```python
from build123d import *

# Parameters (mm, degrees)
SKETCH_1_R           = 1.6
EXTRUDE_1_DEPTH      = 6
SKETCH_2_R           = 30
CUT_EXTRUDE_1_DEPTH  = 13
SKETCH_3_R           = 3.5
CUT_EXTRUDE_2_DEPTH  = 3
SKETCH_5_R           = 2
CUT_EXTRUDE_3_DEPTH  = 23.5
SKETCH_6_R           = 4
CUT_EXTRUDE_4_DEPTH  = 2
CUT_EXTRUDE_6_REACH  = 134
SKETCH_8_W           = 137
SKETCH_8_H           = 2
CUT_EXTRUDE_7_REACH  = 139
SKETCH_9_W           = 1
SKETCH_9_H           = 132
SKETCH_10_W          = 29.336996967
SKETCH_10_H          = 52.898776648
CUT_EXTRUDE_11_DEPTH = 10
SKETCH_11_W          = 8.60940703
SKETCH_11_H          = 108.550160487
CUT_EXTRUDE_12_DEPTH = 10


with BuildPart() as part:
    # 草图1 → 凸台-拉伸1 (new body)
    with BuildSketch(Plane.XY):
        with BuildLine():
            Line((68.5, 66), (20, 66))
            ThreePointArc((20, 66), (0, 46), (-20, 66))
            Line((-20, 66), (-68.5, 66))
            Line((-68.5, 66), (-68.5, 17.384653731))
            ThreePointArc((-68.5, 17.384653731), (-52.74289675, 12.562504398), (-45.954411074, -2.452684221))
            ThreePointArc((-45.954411074, -2.452684221), (-52.74289675, -17.46787284), (-68.5, -22.290022173))
            Line((-68.5, -22.290022173), (-68.5, -66))
            Line((-68.5, -66), (-20, -66))
            ThreePointArc((-20, -66), (0, -46), (20, -66))
            Line((20, -66), (68.5, -66))
            Line((68.5, -66), (68.5, -17.384653731))
            ThreePointArc((68.5, -17.384653731), (45.954411074, 2.452684221), (68.5, 22.290022173))
            Line((68.5, 22.290022173), (68.5, 66))
        make_face()
        with Locations((-63.310606061, -61)):
            Circle(SKETCH_1_R, mode=Mode.SUBTRACT)
        with Locations((63.310606061, -61)):
            Circle(SKETCH_1_R, mode=Mode.SUBTRACT)
        with Locations((-63.310606061, 61)):
            Circle(SKETCH_1_R, mode=Mode.SUBTRACT)
        with Locations((63.310606061, 61)):
            Circle(SKETCH_1_R, mode=Mode.SUBTRACT)
    extrude(amount=EXTRUDE_1_DEPTH)

    # 草图2 → 切除-拉伸1 (cut)
    with BuildSketch(Plane.XY.offset(6)):
        Circle(SKETCH_2_R)
    extrude(amount=-CUT_EXTRUDE_1_DEPTH, mode=Mode.SUBTRACT)

    # 草图3 → 切除-拉伸2 (cut)
    with BuildSketch(Plane(origin=(0, 0, 0), x_dir=(-1, 0, 0), z_dir=(0, 0, -1))):
        with Locations((-63.310606061, 61)):
            Circle(SKETCH_3_R)
        with Locations((63.310606061, 61)):
            Circle(SKETCH_3_R)
        with Locations((-63.310606061, -61)):
            Circle(SKETCH_3_R)
        with Locations((63.310606061, -61)):
            Circle(SKETCH_3_R)
    extrude(amount=-CUT_EXTRUDE_2_DEPTH, mode=Mode.SUBTRACT)

    # 草图5 → 切除-拉伸3 (cut)
    with BuildSketch(Plane.XY.offset(6)):
        with Locations((56.45, 30)):
            Circle(SKETCH_5_R)
        with Locations((-56.45, 30)):
            Circle(SKETCH_5_R)
        with Locations((-56.45, -30)):
            Circle(SKETCH_5_R)
        with Locations((56.45, -30)):
            Circle(SKETCH_5_R)
    extrude(amount=-CUT_EXTRUDE_3_DEPTH, mode=Mode.SUBTRACT)

    # 草图6 → 切除-拉伸4 (cut)
    with BuildSketch(Plane.XY.offset(6)):
        with Locations((56.45, 30)):
            Circle(SKETCH_6_R)
        with Locations((56.45, -30)):
            Circle(SKETCH_6_R)
        with Locations((-56.45, -30)):
            Circle(SKETCH_6_R)
        with Locations((-56.45, 30)):
            Circle(SKETCH_6_R)
    extrude(amount=-CUT_EXTRUDE_4_DEPTH, mode=Mode.SUBTRACT)

    # 草图8 → 切除-拉伸6 (cut, up to next)
    with BuildSketch(Plane(origin=(0, 66, 0), x_dir=(1, 0, 0), z_dir=(0, 1, 0)), mode=Mode.PRIVATE) as cut_extrude_6_sk1:
        with Locations((0, -1)):
            Rectangle(SKETCH_8_W, SKETCH_8_H)
    cut_extrude_6_tool1 = extrude(cut_extrude_6_sk1.sketch, amount=-CUT_EXTRUDE_6_REACH, mode=Mode.PRIVATE) & part.part
    add(cut_extrude_6_tool1.solids().sort_by_distance((0, 66, 1))[0], mode=Mode.SUBTRACT)

    # 草图9 → 切除-拉伸7 (cut, up to next)
    with BuildSketch(Plane(origin=(68.5, 0, 0), x_dir=(0, 0, -1), z_dir=(1, 0, 0)), mode=Mode.PRIVATE) as cut_extrude_7_sk1:
        with Locations((-5.5, 0)):
            Rectangle(SKETCH_9_W, SKETCH_9_H)
    cut_extrude_7_tool1 = extrude(cut_extrude_7_sk1.sketch, amount=-CUT_EXTRUDE_7_REACH, mode=Mode.PRIVATE) & part.part
    add(cut_extrude_7_tool1.solids().sort_by_distance((68.5, 0, 5.5))[0], mode=Mode.SUBTRACT)

    # 草图10 → 切除-拉伸11 (cut)
    with BuildSketch(Plane.XY.offset(5)):
        with Locations((53.831501516, -0.092402659)):
            Rectangle(SKETCH_10_W, SKETCH_10_H)
    extrude(amount=-CUT_EXTRUDE_11_DEPTH, mode=Mode.SUBTRACT)

    # 草图11 → 切除-拉伸12 (cut)
    with BuildSketch(Plane.XY.offset(5)):
        with Locations((64.195296485, 0.655364597)):
            Rectangle(SKETCH_11_W, SKETCH_11_H)
    extrude(amount=-CUT_EXTRUDE_12_DEPTH, mode=Mode.SUBTRACT)


solid = part.part
```
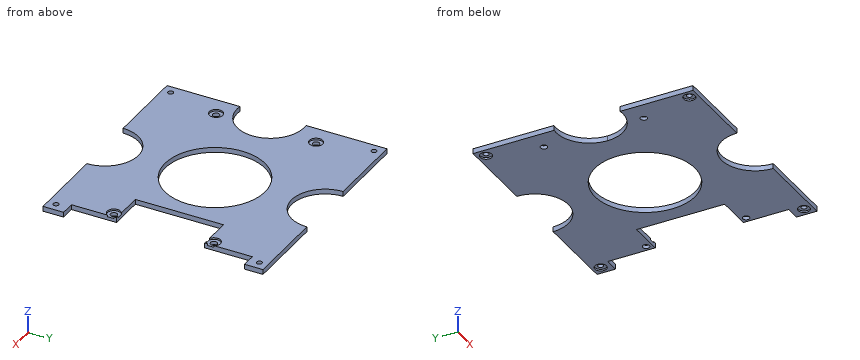
Verification items for the finished model (mm, model axes). Round coordinates to 2 decimals unless told otherwise and drop trailing zeros. Order: outer loops, then holes, each group sorted by start corner. A loop starts at its lowest first (then second) coordinate and runs counter-clockwise, first axis right, second up.
1) Cross-section at C-C, the plane y = 61. Record the cut outline in (x, z), plus the area to 3 significant figures.
Geometry says:
outline: (-68.5, 2) - (-66.81, 2) - (-66.81, 3) - (-64.91, 3) - (-64.91, 5) - (-68.5, 5) - close; (-61.71, 3) - (-59.81, 3) - (-59.81, 2) - (-19.36, 2) - (-19.36, 5) - (-61.71, 5) - close; (19.36, 2) - (59.81, 2) - (59.81, 3) - (61.71, 3) - (61.71, 5) - (19.36, 5) - close; (64.91, 3) - (66.81, 3) - (66.81, 2) - (68.5, 2) - (68.5, 5) - (64.91, 5) - close
area: 268 mm2
2) Cross-section at B-B, the plane y = 14. Record the cut outline in (x, z), plus the area to 3 significant figures.
Geometry says:
outline: (-54.58, 2) - (-26.53, 2) - (-26.53, 5) - (-54.58, 5) - close; (26.53, 2) - (39.16, 2) - (39.16, 5) - (26.53, 5) - close
area: 122 mm2
3) Material ranges on line 1 (Y direction, x = -56.45, z = 2.55); line 2 (Y direction, x = -63, z = 3.8); line 3 (Y direction, x = -1, z = 4.35), recorded low to high.
Geometry says:
line 1: y = -66 to -32, -28 to -20.05, 15.14 to 28, 32 to 66
line 2: y = -66 to -62.57, -59.43 to -22.23, 17.33 to 59.43, 62.57 to 66
line 3: y = -46.03 to -29.98, 29.98 to 46.03
4) Cross-section at D-D, the plane y = -40. Record the cut outline in (x, z), plus the area to 3 significant figures.
Geometry says:
outline: (-68.5, 2) - (59.89, 2) - (59.89, 5) - (-68.5, 5) - close
area: 385 mm2
5) Depth check by flat-ended pin: pin 1 (3 mm diameter, centred on x = -56.45, y = 30, fed in from +Z); pin 2 (7 mm diameter, centred on x = -56.45, y = -30, fed in from +Z). Enter the tip coordinate at first touch or a pass-through.
Geometry says:
pin 1: passes through
pin 2: stops at z = 4
6) Cross-section at A-A, the plane x = 0. Record the cut outline in (y, z).
Geometry says:
outline: (-46, 2) - (-30, 2) - (-30, 5) - (-46, 5) - close; (30, 2) - (46, 2) - (46, 5) - (30, 5) - close
